Could you check a few things on this model? Use its own coordinates, in mm. A direction names the side the tool comes from. Coordinates: 2 decimals unless noted, no trailing zeros. Write each loop counter-clockwise with the first axis right and the second up, starting at its lowest first coordinate (ties: lowest second). Pieces come first, ordered by that corner, then holes. Notation, with made-up numbers: M 56,-36 L 89,-36 A23 cw 89,-12 Z; hole C 60.25,41 d4. An arc over 180 degrees is marked long. Answer as CSV lines item,"result". Start each with the question number.
Item 1: Suppose I cut it at D-D, the plane x = -2. Write out the boundary of the cut face in (y, z).
Item 2: We'd pull the mould along Z, two halves only. Please class faces 5 (the flat face through (0, 15, 35)), 6 (the cylindrical face through (0, -3, 5)), 7 (the flat face through (0, 3, 10)), 8 (the cylindrical face through (-0.54, -2.44, 14.93)): +Z half, -Z half, draft (parallel to the pull), parting line (faces both ways), or undercut.
Item 3: If I drill on line 1 along Z through (x, y) = (1.75, 3.5); line 2 along Z through (x, y) = (-0.5, 2.75); line 3 along Y through (x, z) = (0, 31), over which ranges is the centre line in solid material (lowest first)? Write a range as [from, to].
Item 4: I'm going to push flat-ended pins straight in: P1, Ø2, axis at x = 2, y = 10.5, coming from the -Z side; P2, Ø1, axis at x = -0.5, y = 2.5, coming from the +Z side; P3, Ø0.6, axis at x = -0.5, z = 3.5, coming from the +Y side. Where does each tip first touch, or does it pass through?
Item 5: Suppose I cut it at C-C, the plane z = 10.5. Write out the boundary of the cut face in (x, y), and give its area (3 significant figures).
Item 6: Suppose I cut it at A-A, the plane x = 0. Write out the boundary of the cut face in (y, z).
Item 7: Suppose I cut it at B-B, the plane y = 10. Write out the boundary of the cut face in (x, z), and give its area (3 significant figures).
Item 8: On a 3-axis mill with a long thin cutter (end or side, diameter ignored), from which of +Z, -Z, +X, -X, +Y, -Y can I reach the whole of each face in a straight line? I mean faces 1 (the cylindrical face through (-0.54, 12.56, 29.93)), 2 (the flat face through (1, 3, 5)), 3 (the flat face through (0, 3.997, 5)), 4 (the flat face through (-1, 3, 5)). Say none if no direction works.
```python
from build123d import *

# Parameters (mm, degrees)
SKETCH1_R           = 3
SKETCH1_W           = 2
SKETCH1_H           = 1.993597438
BOSS_EXTRUDE1_DEPTH = 10
SKETCH2_R           = 2.5
BOSS_EXTRUDE2_DEPTH = 10
BOSS_EXTRUDE3_DEPTH = 5
SKETCH4_R           = 2.5
BOSS_EXTRUDE4_DEPTH = 10


with BuildPart() as part:
    # Sketch1 → Boss-Extrude1 (new body)
    with BuildSketch(Plane.XY):
        Circle(SKETCH1_R)
        with Locations((0, 3)):
            Rectangle(SKETCH1_W, SKETCH1_H)
    extrude(amount=BOSS_EXTRUDE1_DEPTH)

    # Sketch2 → Boss-Extrude2 (add)
    with BuildSketch(Plane.XY.offset(10)):
        Circle(SKETCH2_R)
    extrude(amount=BOSS_EXTRUDE2_DEPTH)

    # Sketch3 → Boss-Extrude3 (add)
    with BuildSketch(Plane.XY.offset(20)):
        with BuildLine():
            Line((-3, 0), (-3, 15))
            ThreePointArc((-3, 15), (0, 18), (3, 15))
            Line((3, 15), (3, 0))
            ThreePointArc((3, 0), (0, -3), (-3, 0))
        make_face()
    extrude(amount=BOSS_EXTRUDE3_DEPTH)

    # Sketch4 → Boss-Extrude4 (add)
    with BuildSketch(Plane.XY.offset(25)):
        with Locations((0, 15)):
            Circle(SKETCH4_R)
    extrude(amount=BOSS_EXTRUDE4_DEPTH)


solid = part.part
```
Ans:
1,outline,"M -2.24,0 L 2.24,0 L 2.24,10 L 1.5,10 L 1.5,20 L 17.24,20 L 17.24,25 L 16.5,25 L 16.5,35 L 13.5,35 L 13.5,25 L -2.24,25 L -2.24,20 L -1.5,20 L -1.5,10 L -2.24,10 Z"
2,face 5,"+Z half"
2,face 6,"draft"
2,face 7,"undercut"
2,face 8,"undercut"
3,line 1,"z = [20, 25]"
3,line 2,"z = [0, 10], [20, 25]"
3,line 3,"y = [12.5, 17.5]"
4,P1,"stops at z = 20"
4,P2,"stops at z = 25"
4,P3,"stops at y = 4"
5,outline,"C 0,0 d5"
5,area,"19.6 mm^2"
6,outline,"M -3,0 L 4,0 L 4,10 L 2.5,10 L 2.5,20 L 18,20 L 18,25 L 17.5,25 L 17.5,35 L 12.5,35 L 12.5,25 L -3,25 L -3,20 L -2.5,20 L -2.5,10 L -3,10 Z"
7,outline,"M -3,20 L 3,20 L 3,25 L -3,25 Z"
7,area,"30.0 mm^2"
8,face 1,"+Z"
8,face 2,"-Z, +X, +Y"
8,face 3,"-Z, +X, -X, +Y"
8,face 4,"-Z, -X, +Y"
